Geometry: final body of the model. Coordinates: model frame, mm. Coordinates: 2 decimals unless noted, no trailing zeros. Loops run counter-clockwise (first coordinate to the right, second up) from the corner with the lowest first, then second, coordinate; pieces in that order, holes last. Notation, with made-up numbers: (31, 77.5) - (58, 77.5) arc R24 cw to (58, 96.5) - close; hole circle Ø2 at (67, 53.5). An arc over 180 degrees is marked (long way). Return JSON: item names as keys, results as strings.
from build123d import *

# Parameters (mm, degrees)
SKETCH1_R           = 1.5
BOSS_EXTRUDE1_DEPTH = 6
SKETCH2_R           = 1.5
BOSS_EXTRUDE2_DEPTH = 4
SKETCH3_R           = 1.5
CUT_EXTRUDE1_DEPTH  = 10


with BuildPart() as part:
    # Sketch1 → Boss-Extrude1 (new body)
    with BuildSketch(Plane(origin=(0, 0, 0), x_dir=(1, 0, 0), z_dir=(0, 1, 0))):
        with BuildLine():
            Line((0, 5.230556007), (123.36, 5.230556007))
            ThreePointArc((123.36, 5.230556007), (128.590556007, 0), (123.36, -5.230556007))
            Line((123.36, -5.230556007), (0, -5.230556007))
            ThreePointArc((0, -5.230556007), (-5.230556007, 0), (0, 5.230556007))
        make_face()
        Circle(SKETCH1_R, mode=Mode.SUBTRACT)
        with Locations((123.36, 0)):
            Circle(SKETCH1_R, mode=Mode.SUBTRACT)
    extrude(amount=BOSS_EXTRUDE1_DEPTH)

    # Sketch2 → Boss-Extrude2 (add)
    with BuildSketch(Plane(origin=(0, 6, 0), x_dir=(1, 0, 0), z_dir=(0, 1, 0))):
        with BuildLine():
            Line((3.876609724, 0), (3.876609724, -10))
            ThreePointArc((3.876609724, -10), (0, -13.876609724), (-3.876609724, -10))
            Line((-3.876609724, -10), (-3.876609724, 0))
            ThreePointArc((-3.876609724, 0), (0, 3.876609724), (3.876609724, 0))
        make_face()
        with Locations((0, -10)):
            Circle(SKETCH2_R, mode=Mode.SUBTRACT)
        Circle(SKETCH2_R, mode=Mode.SUBTRACT)
        with BuildLine():
            Line((119.483390276, 0), (119.483390276, -10))
            ThreePointArc((119.483390276, -10), (123.36, -13.876609724), (127.236609724, -10))
            Line((127.236609724, -10), (127.236609724, 0))
            ThreePointArc((127.236609724, 0), (123.36, 3.876609724), (119.483390276, 0))
        make_face()
        with Locations((123.36, 0)):
            Circle(SKETCH2_R, mode=Mode.SUBTRACT)
        with Locations((123.36, -10)):
            Circle(SKETCH2_R, mode=Mode.SUBTRACT)
    extrude(amount=-BOSS_EXTRUDE2_DEPTH)

    # Sketch3 → Cut-Extrude1 (cut)
    with BuildSketch(Plane(origin=(0, 6, 0), x_dir=(1, 0, 0), z_dir=(0, 1, 0))):
        with Locations((51.68, 0)):
            Circle(SKETCH3_R)
        with Locations((71.68, 0)):
            Circle(SKETCH3_R)
    extrude(amount=-CUT_EXTRUDE1_DEPTH, mode=Mode.SUBTRACT)


solid = part.part
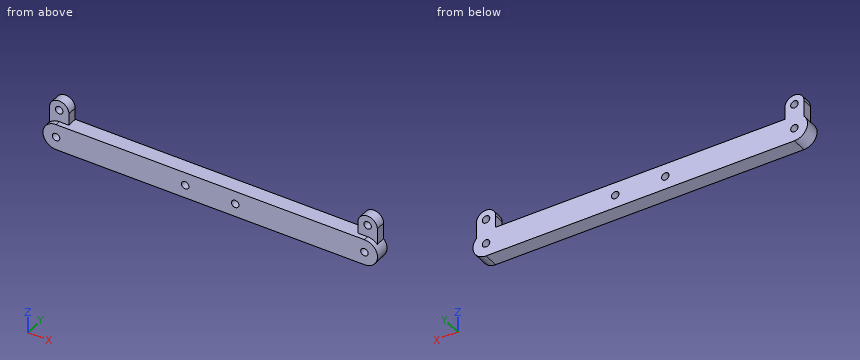
Item 1: Ray query, probe 1 along X at (y, z) = (3.55, 0); probe 2 along X at (y, z) = (3.75, 10); probe 3 along Z at (x, y) = (0, 4.6). Return the intervals inside material, ascending. Write a range as from..to.
Worked out:
{"probe 1": "-5.23..-1.5, 1.5..50.18, 53.18..70.18, 73.18..121.86, 124.86..128.59", "probe 2": "-3.88..-1.5, 1.5..3.88, 119.48..121.86, 124.86..127.24", "probe 3": "-5.23..-1.5, 1.5..8.5, 11.5..13.88"}
Item 2: First-contact query: pin 1 Ø3.5 at (x, z) = (0, 10) entering from -Y; pin 2 Ø3 at (y, z) = (3, 8.5) entering from -X; pin 3 Ø2 at (y, z) = (4.5, 8.5) entering from +X. Flat tips, straight axial feed; report the tip coordinate or a pass-through.
Worked out:
{"pin 1": "y = 2", "pin 2": "x = -3.88", "pin 3": "x = 127.24"}
Item 3: Section query D-D, the plane z = -4. Return loops of the section in (x, y).
Worked out:
{"outline": "(-3.37, 0) - (126.73, 0) - (126.73, 6) - (-3.37, 6) - close"}
Item 4: Section query A-A, the plane x = 51.68. Return loops of the section in (y, z), and give its area (3 significant figures).
Worked out:
{"outline": "(0, -5.23) - (6, -5.23) - (6, -1.5) - (0, -1.5) - close; (0, 1.5) - (6, 1.5) - (6, 5.23) - (0, 5.23) - close", "area": "44.8 mm^2"}
Item 5: Section query B-B, the plane y = 4.15. Return loops of the section in (x, z), and give its area (3 significant figures).
Worked out:
{"outline": "(-3.88, 3.51) arc R5.23 ccw to (0, -5.23) - (123.36, -5.23) arc R5.23 ccw to (127.24, 3.51) - (127.24, 10) arc R3.88 ccw to (119.48, 10) - (119.48, 5.23) - (3.88, 5.23) - (3.88, 10) arc R3.88 ccw to (-3.88, 10) - close; hole circle Ø3 at (0, 0); hole circle Ø3 at (0, 10); hole circle Ø3 at (51.68, 0); hole circle Ø3 at (71.68, 0); hole circle Ø3 at (123.36, 0); hole circle Ø3 at (123.36, 10)", "area": "1,460 mm^2"}
Item 6: Section query C-C, the plane x = 7. Return loops of the section in (y, z), and give its area (3 significant figures).
Worked out:
{"outline": "(0, -5.23) - (6, -5.23) - (6, 5.23) - (0, 5.23) - close", "area": "62.8 mm^2"}
